```python
from build123d import *

# Parameters (mm, degrees)
SKETCH_1_W          = 160
SKETCH_1_H          = 98
EXTRUDE_1_DEPTH     = 39
SKETCH_2_W          = 97
SKETCH_2_H          = 29
CUT_EXTRUDE_1_DEPTH = 15
SKETCH_3_R          = 1.75
CUT_EXTRUDE_2_DEPTH = 5
SKETCH_4_R          = 1.75
CUT_EXTRUDE_3_DEPTH = 5
SKETCH_5_W          = 8
SKETCH_5_H          = 9
CUT_EXTRUDE_4_DEPTH = 9


with BuildPart() as part:
    # 草图1 → 拉伸1 (new body)
    with BuildSketch(Plane(origin=(0, 0, 0), x_dir=(1, 0, 0), z_dir=(0, 1, 0))):
        Rectangle(SKETCH_1_W, SKETCH_1_H)
    extrude(amount=EXTRUDE_1_DEPTH)

    # 草图2 → 切除-拉伸1 (cut)
    with BuildSketch(Plane(origin=(80, 0, 0), x_dir=(0, 0, -1), z_dir=(1, 0, 0))):
        with Locations((-0.5, 24.5)):
            Rectangle(SKETCH_2_W, SKETCH_2_H)
    extrude(amount=-CUT_EXTRUDE_1_DEPTH, mode=Mode.SUBTRACT)

    # 草图3 → 切除-拉伸2 (cut)
    with BuildSketch(Plane(origin=(0, 0, -49), x_dir=(-1, 0, 0), z_dir=(0, 0, -1))):
        with Locations((-59, 28.5)):
            Circle(SKETCH_3_R)
        with Locations((73.5, 28.5)):
            Circle(SKETCH_3_R)
        with Locations((58, 19)):
            Circle(SKETCH_3_R)
        with Locations((-59, 10.5)):
            Circle(SKETCH_3_R)
        with BuildLine():
            Line((-76.5, 30.25), (-80, 30.25))
            Line((-80, 30.25), (-80, 26.75))
            Line((-80, 26.75), (-76.5, 26.75))
            ThreePointArc((-76.5, 26.75), (-74.75, 28.5), (-76.5, 30.25))
        make_face()
    extrude(amount=-CUT_EXTRUDE_2_DEPTH, mode=Mode.SUBTRACT)

    # 草图4 → 切除-拉伸3 (cut)
    with BuildSketch(Plane.XZ):
        with Locations(Location((22, -16, 0), (0, 0, 270))):
            Circle(SKETCH_4_R)
        with Locations(Location((22, 16, 0), (0, 0, 270))):
            Circle(SKETCH_4_R)
        with Locations(Location((-56, -16, 0), (0, 0, 270))):
            Circle(SKETCH_4_R)
        with Locations(Location((-56, 16, 0), (0, 0, 270))):
            Circle(SKETCH_4_R)
        with Locations(Location((-75.5, 43.5, 0), (0, 0, 270))):
            Circle(SKETCH_4_R)
        with BuildLine():
            Line((76.5, -43.75), (80, -43.75))
            Line((80, -43.75), (80, -40.25))
            Line((80, -40.25), (76.5, -40.25))
            ThreePointArc((76.5, -40.25), (74.75, -42), (76.5, -43.75))
        make_face()
    extrude(amount=-CUT_EXTRUDE_3_DEPTH, mode=Mode.SUBTRACT)

    # 草图5 → 切除-拉伸4 (cut)
    with BuildSketch(Plane(origin=(0, 10, 0), x_dir=(-1, 0, 0), z_dir=(0, 1, 0))):
        with Locations((-76, -43.5)):
            Rectangle(SKETCH_5_W, SKETCH_5_H)
    extrude(amount=-CUT_EXTRUDE_4_DEPTH, mode=Mode.SUBTRACT)


solid = part.part
```
Part model, mm, in its own coordinate system. A direction names the side the tool comes from. Round coordinates to 2 decimals unless told otherwise and drop trailing zeros. Loops run counter-clockwise (first coordinate to the right, second up) from the corner with the lowest first, then second, coordinate; pieces in that order, holes last.
Item 1: Mould opens along Y. For faces 1 (the face through (-57.55, 2.46, 15.19)), 2 (the face through (57.383, 27.83, -46.535)), 3 (the face through (-1, 0, -1)) say: +Y half, -Y half, draft (parallel to the pull), parting line (faces both ways), or undercut.
Item 2: Drill centre lines: line 1 (Y direction, x = -73.5, z = -46.85); line 2 (Y direction, x = 59, z = -45); line 3 (X direction, y = 3, z = 16). Where is each one in solid material? Low to high.
Item 3: Cut at A-A, the plane y = 19. Give the cut face in (x, z).
Item 4: Cut at D-D, the plane z = -16. Give the cut face in (x, y).
Item 5: Cut at B-B, the plane z = 35.5. Give the cut face in (x, y).
Item 6: Drop flat-ended pins along their axis: P1, Ø1, axis at x = -56, z = -15.5, coming from the -Y side; P2, Ø1, axis at x = 59, y = 9.5, coming from the -Z side; P3, Ø2.5, axis at y = 7, z = -41.5, coming from the +X side; P4, Ø12, axis at x = 75.5, y = 14.5, coming from the +Z side. Give the stop position or say it passes through.
Item 7: 3-axis set-ups, long thin cutter, end or side, ignore diameter. For faces 4 (the face through (76, 6, -39)), 5 (the face through (59, 11, -44)), 6 (the face through (73, 10, 1)), 7 (the face through (22, 5, -16)): which of +Z, -Z, +X, -X, +Y, -Y reach the whole face in a straight line?
Item 8: Cut at C-C, the plane y = 28.5. Give the cut face in (x, z), then the cut area to 3 significant figures.
A:
1. face 1: draft
1. face 2: undercut
1. face 3: -Y half
2. line 1: y = 0 to 26.75, 30.25 to 39
2. line 2: y = 0 to 8.75, 12.25 to 26.75, 30.25 to 39
2. line 3: x = -80 to -57.75, -54.25 to 20.25, 23.75 to 80
3. outline: (-80, -49) - (-59.75, -49) - (-59.75, -44) - (-56.25, -44) - (-56.25, -49) - (80, -49) - (80, -48) - (65, -48) - (65, 49) - (-80, 49) - close
4. outline: (-80, 0) - (-57.75, 0) - (-57.75, 5) - (-54.25, 5) - (-54.25, 0) - (20.25, 0) - (20.25, 5) - (23.75, 5) - (23.75, 0) - (80, 0) - (80, 10) - (65, 10) - (65, 39) - (-80, 39) - close
5. outline: (-80, 0) - (80, 0) - (80, 10) - (65, 10) - (65, 39) - (-80, 39) - close
6. P1: stops at y = 5
6. P2: stops at z = -44
6. P3: stops at x = 72
6. P4: stops at z = 49
7. face 4: +X, +Y
7. face 5: -Z
7. face 6: +Z, +X, +Y
7. face 7: -Y
8. outline: (-80, -49) - (-75.25, -49) - (-75.25, -44) - (-71.75, -44) - (-71.75, -49) - (57.25, -49) - (57.25, -44) - (60.75, -44) - (60.75, -49) - (74.75, -49) - (74.75, -48) - (65, -48) - (65, 49) - (-80, 49) - close
8. area: 14,200 mm2
